Check sheet for the modelled part. Datum: model origin and axes. Units: mm. A direction names the side the tool comes from. Round coordinates to 2 decimals unless told otherwise and drop trailing zeros. Order: outer loops, then holes, each group sorted by start corner. A loop starts at its lowest first (then second) coordinate and runs counter-clockwise, first axis right, second up. Notation, with made-up numbers: (11.5, 26) -> (19.5, 26) arc R32 ccw to (19.5, 60) -> close; hole circle Ø4 at (-39, -28). An arc over 180 degrees is marked (long way). Answer in a Markdown table with one row per item.
from build123d import *

# Parameters (mm, degrees)
SKETCH_1_W          = 60
SKETCH_1_H          = 60
EXTRUDE_1_DEPTH     = 30
SKETCH_2_R          = 1.75
CUT_EXTRUDE_1_DEPTH = 30
SKETCH_3_R          = 12.5
CUT_EXTRUDE_2_DEPTH = 3
SKETCH_4_W          = 20
SKETCH_4_H          = 20
CUT_EXTRUDE_3_DEPTH = 3
FILLET_1_R          = 5


with BuildPart() as part:
    # 草图1 → 凸台-拉伸1 (new body)
    with BuildSketch(Plane(origin=(0, 0, 0), x_dir=(1, 0, 0), z_dir=(0, 1, 0))):
        Rectangle(SKETCH_1_W, SKETCH_1_H)
    extrude(amount=EXTRUDE_1_DEPTH)

    # 草图2 → 切除-拉伸1 (cut)
    with BuildSketch(Plane(origin=(0, 30, 0), x_dir=(1, 0, 0), z_dir=(0, 1, 0))):
        with Locations(Location((25, 25, 0), (0, 0, 270))):
            Circle(SKETCH_2_R)
        with Locations(Location((-25, 25, 0), (0, 0, 270))):
            Circle(SKETCH_2_R)
        with Locations(Location((-25, -25, 0), (0, 0, 270))):
            Circle(SKETCH_2_R)
        with Locations(Location((25, -25, 0), (0, 0, 270))):
            Circle(SKETCH_2_R)
    extrude(amount=-CUT_EXTRUDE_1_DEPTH, mode=Mode.SUBTRACT)

    # 草图3 → 切除-拉伸2 (cut)
    with BuildSketch(Plane(origin=(0, 30, 0), x_dir=(1, 0, 0), z_dir=(0, 1, 0))):
        with Locations(Location((0, 0, 0), (0, 0, 270))):
            Circle(SKETCH_3_R)
    extrude(amount=-CUT_EXTRUDE_2_DEPTH, mode=Mode.SUBTRACT)

    # 草图4 → 切除-拉伸3 (cut)
    with BuildSketch(Plane.XZ):
        Rectangle(SKETCH_4_W, SKETCH_4_H)
    extrude(amount=-CUT_EXTRUDE_3_DEPTH, mode=Mode.SUBTRACT)

    # 圆角1
    fillet_1_edges = [part.edges().sort_by_distance(p)[0] for p in [
        (30, 15, 30),
        (-30, 15, 30),
        (-30, 15, -30),
        (30, 15, -30),
    ]]
    fillet(fillet_1_edges, radius=FILLET_1_R)


solid = part.part
Item 1: Mould release check, pull along Z, two halves, no side actions. Record for faces 1 (the flat face through (0, 15, 30)), 2 (the cylindrical face through (-29, 15, -28)), 3 (the cylindrical face through (-23.265, 15.21, 24.772)): pulls with the +Z half, pulls with the -Z half, needs draft (parallel to the pull), parting line crosses it, or undercut.
Result sheet:
| item | result |
|---|---|
| face 1 | pulls with the +Z half |
| face 2 | pulls with the -Z half |
| face 3 | undercut |
Item 2: Cross-section at B-B (z = 0). Record the boundary of the cut face in (x, y).
Result sheet:
| item | result |
|---|---|
| outline | (-30, 0) -> (-10, 0) -> (-10, 3) -> (10, 3) -> (10, 0) -> (30, 0) -> (30, 30) -> (12.5, 30) -> (12.5, 27) -> (-12.5, 27) -> (-12.5, 30) -> (-30, 30) -> close |
Item 3: Scan lines: line 1 (X direction, y = 14.75, z = 25); line 2 (Y direction, x = 6, z = 0.5); line 3 (X direction, y = 28, z = -7). Record each from-to range of solid material in increasing order. Write a range as [from, to].
Result sheet:
| item | result |
|---|---|
| line 1 | x = [-30, -26.75], [-23.25, 23.25], [26.75, 30] |
| line 2 | y = [3, 27] |
| line 3 | x = [-30, -10.36], [10.36, 30] |
Item 4: Cross-section at A-A (y = 18.5). Record the boundary of the cut face in (x, z).
Result sheet:
| item | result |
|---|---|
| outline | (-30, -25) arc R5 ccw to (-25, -30) -> (25, -30) arc R5 ccw to (30, -25) -> (30, 25) arc R5 ccw to (25, 30) -> (-25, 30) arc R5 ccw to (-30, 25) -> close; hole circle Ø3.5 at (-25, -25); hole circle Ø3.5 at (-25, 25); hole circle Ø3.5 at (25, -25); hole circle Ø3.5 at (25, 25) |
Item 5: Depth check by flat-ended pin: P1, Ø12.5, axis at x = 2.5, z = -5, coming from the +Y side. Enter the tip coordinate at first touch or a pass-through.
Result sheet:
| item | result |
|---|---|
| P1 | stops at y = 27 |
Item 6: Set-up check for faces 4 (the flat face through (-10, 1, 0)), 5 (the cylindrical face through (3.755, 28.521, 11.923)), 6 (the cylindrical face through (-29, 15, 28)): record each of +Z, -Z, +X, -X, +Y, -Y from which the full face is reachable in a straight line by a thin tool's end or side.
Result sheet:
| item | result |
|---|---|
| face 4 | -Y |
| face 5 | +Y |
| face 6 | +Z, -X, +Y, -Y |
Item 7: Cross-section at C-C (z = -6.5). Record the boundary of the cut face in (x, y), and give its area (3 significant figures).
Result sheet:
| item | result |
|---|---|
| outline | (-30, 0) -> (-10, 0) -> (-10, 3) -> (10, 3) -> (10, 0) -> (30, 0) -> (30, 30) -> (10.68, 30) -> (10.68, 27) -> (-10.68, 27) -> (-10.68, 30) -> (-30, 30) -> close |
| area | 1,680 mm^2 |
